Answer from the drawing. Dimensions are ordinates in mm from the lowest x, y and z of the part. A direction names the side the tool comes from. Give positions to 0.01 mm unless a question says otherwise; leave off trailing zeros. Order: outer loops, then holes, each group sorted by start corner. A loop starts at its lowest first (then second) coordinate and runs counter-clockwise, first axis right, second up. Notation, with made-up numbers: (-40, 8) - (-27, 8) arc R19 ccw to (-27, 24) - close; hole circle Ø11 at (-22.5, 58.25). An arc over 180 degrees is marked (long way). Use a Markdown table: item, result. Add a question column.
1) Find section A-A, the plane y = 3.81. Determine the outline of the cut face in (x, z) (3 decimals), plus the area to 3 significant figures.
2) Find section B-B, the plane z = 2.6. Determine the outline of the cut face in (x, y) (3 decimals).
3) For the marked faces 1 and 2, determine the directions among +Z, -Z, +X, -X, +Y, -Y from which every point of the face is accessible in a straight line to the end or side of a thin tool.
4) Straight lines are drawn through the part: line 1 (Y direction, x = 8.75, z = 3.05); line 2 (X direction, y = 40, z = 1.3); line 3 (Y direction, x = 14.75, z = 1.6). For each, find the intervals that lie inside material, in ascending order.
5) Find section C-C, the plane y = 40.5. Determine the outline of the cut face in (x, z).
6) Flat-ended cylindrical pins translate along their axes: pin 1 (2 mm diameter, centred on y = 6.5, z = 4, fed in from -X); pin 2 (2 mm diameter, centred on x = 14.525, y = 3.81, fed in from -Z). Find the tip coordinate at first contact, or state that the pin passes through.
7) The mould has two halves that part along X. Classify the marked faces 3, 4 and 5: released by +X, released by -X, zero draft, split by the parting line, or undercut.
8) Find section D-D, the plane x = 11.5. Determine the outline of the cut face in (y, z).
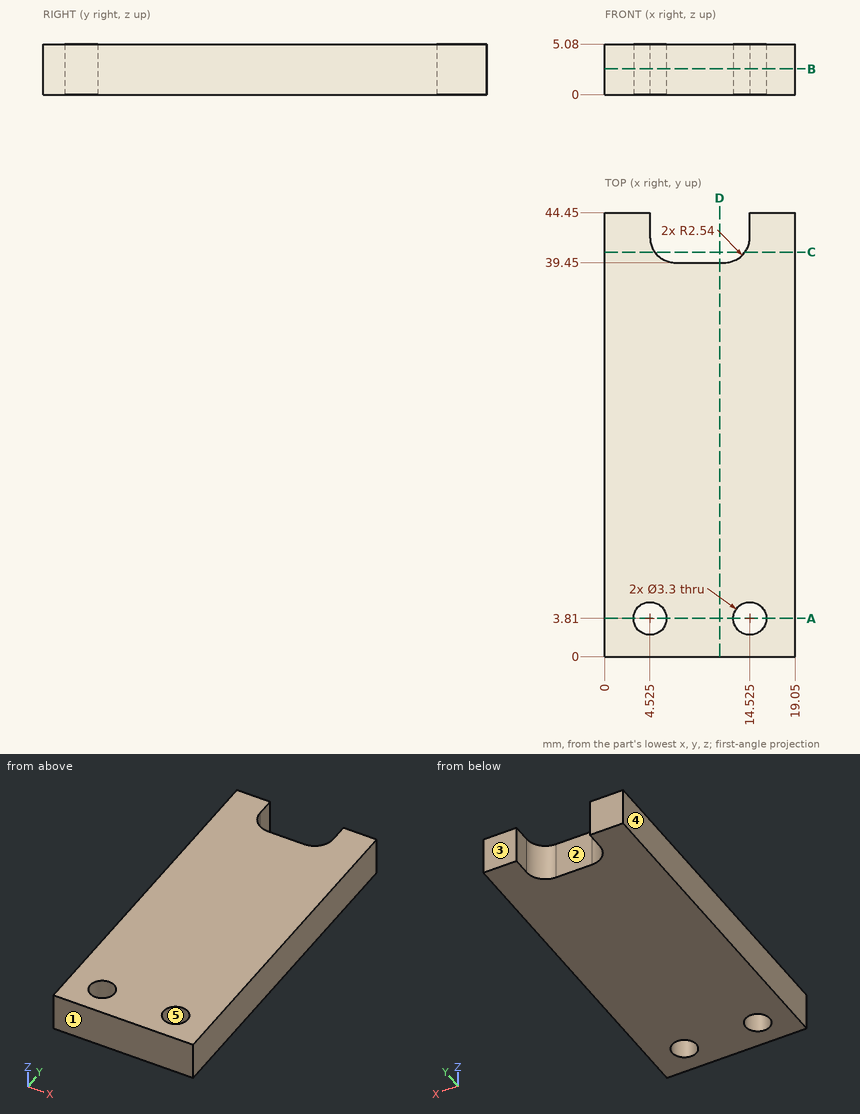
The answers:
| question | item | result |
|---|---|---|
| 1 | outline | (0, 0) - (2.875, 0) - (2.875, 5.08) - (0, 5.08) - close; (6.175, 0) - (12.875, 0) - (12.875, 5.08) - (6.175, 5.08) - close; (16.175, 0) - (19.05, 0) - (19.05, 5.08) - (16.175, 5.08) - close |
| 1 | area | 63.2 mm2 |
| 2 | outline | (0, 0) - (19.05, 0) - (19.05, 44.45) - (14.525, 44.45) - (14.525, 41.99) arc R2.54 cw to (11.985, 39.45) - (7.065, 39.45) arc R2.54 cw to (4.525, 41.99) - (4.525, 44.45) - (0, 44.45) - close; hole circle Ø3.3 at (4.525, 3.81); hole circle Ø3.3 at (14.525, 3.81) |
| 3 | face 1 | +Z, -Z, +X, -X, -Y |
| 3 | face 2 | +Z, -Z, +Y |
| 4 | line 1 | 0 to 39.45 |
| 4 | line 2 | 0 to 5.49, 13.56 to 19.05 |
| 4 | line 3 | 0 to 2.18, 5.44 to 44.45 |
| 5 | outline | (0, 0) - (5.01, 0) - (5.01, 5.08) - (0, 5.08) - close; (14.04, 0) - (19.05, 0) - (19.05, 5.08) - (14.04, 5.08) - close |
| 6 | pin 1 | x = 0 |
| 6 | pin 2 | through |
| 7 | face 3 | zero draft |
| 7 | face 4 | released by -X |
| 7 | face 5 | undercut |
| 8 | outline | (0, 0) - (39.45, 0) - (39.45, 5.08) - (0, 5.08) - close |
